```python
from build123d import *

# Parameters (mm, degrees)
SKETCH1_R           = 2.4892
SKETCH1_R_2         = 2.54
BOSS_EXTRUDE1_DEPTH = 3.175
BOSS_EXTRUDE2_START = -3.175
SKETCH3_R           = 2.4892
BOSS_EXTRUDE2_DEPTH = 3.175
SKETCH4_R           = 2.4892
CUT_EXTRUDE1_DEPTH  = 122.275025768


with BuildPart() as part:
    # Sketch1 → Boss-Extrude1 (new body)
    with BuildSketch(Plane(origin=(0, 0, 0), x_dir=(1, 0, 0), z_dir=(0, 1, 0))):
        with BuildLine():
            Line((0, 63.5), (-33.02, 63.5))
            ThreePointArc((-33.02, 63.5), (-36.612102448, 64.987897552), (-38.1, 68.58))
            Line((-38.1, 68.58), (-38.1, 77.47))
            ThreePointArc((-38.1, 77.47), (-36.612102448, 81.062102448), (-33.02, 82.55))
            Line((-33.02, 82.55), (77.47, 82.55))
            ThreePointArc((77.47, 82.55), (81.062102448, 81.062102448), (82.55, 77.47))
            Line((82.55, 77.47), (82.55, -33.02))
            ThreePointArc((82.55, -33.02), (81.062102448, -36.612102448), (77.47, -38.1))
            Line((77.47, -38.1), (68.58, -38.1))
            ThreePointArc((68.58, -38.1), (64.987897552, -36.612102448), (63.5, -33.02))
            Line((63.5, -33.02), (63.5, 0))
            ThreePointArc((63.5, 0), (44.901280605, 44.901280605), (0, 63.5))
        make_face()
        with Locations(Location((-28.575, 73.025, 0), (0, 0, 270))):
            Circle(SKETCH1_R, mode=Mode.SUBTRACT)
        with Locations(Location((-15.875, 73.025, 0), (0, 0, 270))):
            Circle(SKETCH1_R, mode=Mode.SUBTRACT)
        with Locations(Location((-3.175, 73.025, 0), (0, 0, 270))):
            Circle(SKETCH1_R, mode=Mode.SUBTRACT)
        with Locations(Location((9.525, 73.025, 0), (0, 0, 270))):
            Circle(SKETCH1_R, mode=Mode.SUBTRACT)
        with Locations(Location((22.225, 73.025, 0), (0, 0, 270))):
            Circle(SKETCH1_R, mode=Mode.SUBTRACT)
        with Locations(Location((34.925, 73.025, 0), (0, 0, 270))):
            Circle(SKETCH1_R, mode=Mode.SUBTRACT)
        with Locations(Location((47.625, 73.025, 0), (0, 0, 270))):
            Circle(SKETCH1_R, mode=Mode.SUBTRACT)
        with Locations(Location((60.325, 73.025, 0), (0, 0, 270))):
            Circle(SKETCH1_R, mode=Mode.SUBTRACT)
        with Locations(Location((73.025, 73.025, 0), (0, 0, 270))):
            Circle(SKETCH1_R, mode=Mode.SUBTRACT)
        with Locations(Location((73.025, 60.325, 0), (0, 0, 270))):
            Circle(SKETCH1_R, mode=Mode.SUBTRACT)
        with Locations(Location((73.025, 47.625, 0), (0, 0, 270))):
            Circle(SKETCH1_R, mode=Mode.SUBTRACT)
        with Locations(Location((73.025, 34.925, 0), (0, 0, 270))):
            Circle(SKETCH1_R, mode=Mode.SUBTRACT)
        with Locations(Location((73.025, 22.225, 0), (0, 0, 270))):
            Circle(SKETCH1_R, mode=Mode.SUBTRACT)
        with Locations(Location((73.025, 9.525, 0), (0, 0, 270))):
            Circle(SKETCH1_R, mode=Mode.SUBTRACT)
        with Locations(Location((73.025, -3.175, 0), (0, 0, 270))):
            Circle(SKETCH1_R, mode=Mode.SUBTRACT)
        with Locations(Location((73.025, -15.875, 0), (0, 0, 270))):
            Circle(SKETCH1_R, mode=Mode.SUBTRACT)
        with Locations(Location((73.025, -28.575, 0), (0, 0, 270))):
            Circle(SKETCH1_R, mode=Mode.SUBTRACT)
        with Locations(Location((50.8, 50.8, 0), (0, 0, 270))):
            Circle(SKETCH1_R_2, mode=Mode.SUBTRACT)
    extrude(amount=BOSS_EXTRUDE1_DEPTH)

    # Sketch3 → Boss-Extrude2 (add)
    with BuildSketch(Plane(origin=(0, 3.175, 0), x_dir=(1, 0, 0), z_dir=(0, 1, 0)).offset(BOSS_EXTRUDE2_START)):
        with BuildLine():
            ThreePointArc((-33.02, 63.5), (-35.859806331, 64.367886516), (-37.729286039, 66.675))
            ThreePointArc((-37.729286039, 66.675), (-38.006460322, 67.609632307), (-38.1, 68.58))
            Line((-38.1, 68.58), (-38.1, 77.47))
            ThreePointArc((-38.1, 77.47), (-36.612102448, 81.062102448), (-33.02, 82.55))
            Line((-33.02, 82.55), (77.47, 82.55))
            ThreePointArc((77.47, 82.55), (81.062102448, 81.062102448), (82.55, 77.47))
            Line((82.55, 77.47), (82.55, -33.02))
            ThreePointArc((82.55, -33.02), (81.062102448, -36.612102448), (77.47, -38.1))
            Line((77.47, -38.1), (68.58, -38.1))
            ThreePointArc((68.58, -38.1), (67.609632307, -38.006460322), (66.675, -37.729286039))
            ThreePointArc((66.675, -37.729286039), (64.367886516, -35.859806331), (63.5, -33.02))
            Line((63.5, -33.02), (63.5, -39.37))
            ThreePointArc((63.5, -39.37), (64.987897552, -42.962102448), (68.58, -44.45))
            Line((68.58, -44.45), (80.645, -44.45))
            ThreePointArc((80.645, -44.45), (84.237102448, -42.962102448), (85.725, -39.37))
            Line((85.725, -39.37), (85.725, 80.645))
            ThreePointArc((85.725, 80.645), (84.237102448, 84.237102448), (80.645, 85.725))
            Line((80.645, 85.725), (-39.37, 85.725))
            ThreePointArc((-39.37, 85.725), (-42.962102448, 84.237102448), (-44.45, 80.645))
            Line((-44.45, 80.645), (-44.45, 68.58))
            ThreePointArc((-44.45, 68.58), (-42.962102448, 64.987897552), (-39.37, 63.5))
            Line((-39.37, 63.5), (-33.02, 63.5))
        make_face()
        with Locations((73.025, -28.575)):
            Circle(SKETCH3_R)
        with Locations((73.025, -15.875)):
            Circle(SKETCH3_R)
        with Locations((73.025, -3.175)):
            Circle(SKETCH3_R)
        with Locations((73.025, 9.525)):
            Circle(SKETCH3_R)
        with Locations((73.025, 22.225)):
            Circle(SKETCH3_R)
        with Locations((73.025, 34.925)):
            Circle(SKETCH3_R)
        with Locations((73.025, 47.625)):
            Circle(SKETCH3_R)
        with Locations((73.025, 60.325)):
            Circle(SKETCH3_R)
        with Locations((73.025, 73.025)):
            Circle(SKETCH3_R)
        with Locations((60.325, 73.025)):
            Circle(SKETCH3_R)
        with Locations((47.625, 73.025)):
            Circle(SKETCH3_R)
        with Locations((34.925, 73.025)):
            Circle(SKETCH3_R)
        with Locations((22.225, 73.025)):
            Circle(SKETCH3_R)
        with Locations((9.525, 73.025)):
            Circle(SKETCH3_R)
        with Locations((-3.175, 73.025)):
            Circle(SKETCH3_R)
        with Locations((-15.875, 73.025)):
            Circle(SKETCH3_R)
        with Locations((-28.575, 73.025)):
            Circle(SKETCH3_R)
    extrude(amount=BOSS_EXTRUDE2_DEPTH)

    # Sketch4 → Cut-Extrude1 (cut, through all)
    with BuildSketch(Plane(origin=(0, 3.175, 0), x_dir=(1, 0, 0), z_dir=(0, 1, 0))):
        with Locations(Location((63.5, 76.2, 0), (0, 0, 270))):
            Circle(SKETCH4_R)
        with Locations(Location((76.2, 76.2, 0), (0, 0, 270))):
            Circle(SKETCH4_R)
        with Locations(Location((76.2, 63.5, 0), (0, 0, 270))):
            Circle(SKETCH4_R)
        with Locations(Location((76.2, 50.8, 0), (0, 0, 270))):
            Circle(SKETCH4_R)
        with Locations(Location((76.2, 38.1, 0), (0, 0, 270))):
            Circle(SKETCH4_R)
        with Locations(Location((50.8, 76.2, 0), (0, 0, 270))):
            Circle(SKETCH4_R)
        with Locations(Location((38.1, 76.2, 0), (0, 0, 270))):
            Circle(SKETCH4_R)
        with Locations(Location((25.4, 76.2, 0), (0, 0, 270))):
            Circle(SKETCH4_R)
        with Locations(Location((76.2, -25.4, 0), (0, 0, 270))):
            Circle(SKETCH4_R)
        with Locations(Location((76.2, -12.7, 0), (0, 0, 270))):
            Circle(SKETCH4_R)
        with Locations(Location((76.2, 0, 0), (0, 0, 270))):
            Circle(SKETCH4_R)
        with Locations(Location((76.2, 12.7, 0), (0, 0, 270))):
            Circle(SKETCH4_R)
        with Locations(Location((76.2, 25.4, 0), (0, 0, 270))):
            Circle(SKETCH4_R)
        with Locations(Location((12.7, 76.2, 0), (0, 0, 270))):
            Circle(SKETCH4_R)
        with Locations(Location((0, 76.2, 0), (0, 0, 270))):
            Circle(SKETCH4_R)
        with Locations(Location((-12.7, 76.2, 0), (0, 0, 270))):
            Circle(SKETCH4_R)
        with Locations(Location((-38.1, 76.2, 0), (0, 0, 270))):
            Circle(SKETCH4_R)
        with Locations(Location((-25.4, 76.2, 0), (0, 0, 270))):
            Circle(SKETCH4_R)
        with Locations(Location((76.2, -38.1, 0), (0, 0, 270))):
            Circle(SKETCH4_R)
    extrude(amount=-CUT_EXTRUDE1_DEPTH, mode=Mode.SUBTRACT)


solid = part.part
```
Geometry: final body of the model. Coordinates: model frame, mm. Give positions to 0.01 mm unless a question says otherwise; leave off trailing zeros. Write each loop counter-clockwise with the first axis right and the second up, starting at its lowest first coordinate (ties: lowest second). Pieces come first, ordered by that corner, then holes.
1. Line query: probe 1 along X at (y, z) = (2.05, 25.4) (3 decimals); probe 2 along X at (y, z) = (2.25, -51) (3 decimals); probe 3 along X at (y, z) = (2.65, -65) (3 decimals). Output: solid intervals per line, ascending.
2. Draft query along Z for faces 1 (the cylindrical face through (74.69, 1.61, 36.12)), 2 (the cylindrical face through (64.949, 1.565, 42.922)), 3 (the flat face through (49, 0, -45)). Return one class per face: released by +Z, released by -Z, zero draft, split by the parting line, or undercut.
3. Section query D-D, the plane x = 38.1. Return loops of the section in (y, z) (3 decimals).
4. Pin query (flat end, axial travel): P1, Ø3, axis at x = 76.2, z = 0, coming from the -Y side; P2, Ø1.5, axis at x = 34, y = 2.5, coming from the +Z side; P3, Ø1.5, axis at y = 2.5, z = -19.5, coming from the -X side. Return the tip coordinate at first contact, or that it passes through.
5. Section query B-B, the plane x = -25.4. Return loops of the section in (y, z) (3 decimals), then the cut area to 3 significant figures.
6. Section query C-C, the plane y = 1.5. Count the separate pieces of the cut face and the enclosed holes in it, then the cut area to 3 significant figures.
7. Section query A-A, the plane z = -50.8. Return loops of the section in (x, y) (3 decimals).
Computed:
1. probe 1: x = 63.5 to 73.711, 78.689 to 85.725
1. probe 2: x = 37.832 to 48.268, 53.332 to 73.719, 78.681 to 85.725
1. probe 3: x = -42.974 to 74.214, 78.186 to 85.725
2. face 1: undercut
2. face 2: released by +Z
2. face 3: zero draft
3. outline: (0, -85.725) - (3.175, -85.725) - (3.175, -78.689) - (0, -78.689) - close; (0, -73.711) - (3.175, -73.711) - (3.175, -50.8) - (0, -50.8) - close
4. P1: passes through
4. P2: stops at z = -53.15
4. P3: stops at x = 60.18
5. outline: (0, -85.725) - (3.175, -85.725) - (3.175, -78.689) - (0, -78.689) - close; (0, -73.711) - (3.175, -73.711) - (3.175, -63.5) - (0, -63.5) - close
5. area: 54.8 mm2
6. separate pieces: 1
6. enclosed holes: 20
6. area: 5,740 mm2
7. outline: (38.1, 0) - (48.26, 0) - (48.26, 3.175) - (38.1, 3.175) - close; (53.34, 0) - (73.711, 0) - (73.711, 3.175) - (53.34, 3.175) - close; (78.689, 0) - (85.725, 0) - (85.725, 3.175) - (78.689, 3.175) - close
